The model under review builds one solid part; all positions refer to its coordinate system, in mm. A direction names the side the tool comes from. Coordinates: 2 decimals unless noted, no trailing zeros. Order: outer loops, then holes, each group sorted by start corner. A loop starts at its lowest first (then second) coordinate and runs counter-clockwise, first axis right, second up. Notation, with made-up numbers: (6.5, -30.5) -> (35.5, -30.5) arc R19 ccw to (35.5, 3.5) -> close; hole circle Ø8 at (24, -10.75). An arc over 180 degrees is marked (long way). Put each result on its own line as item: value.
from build123d import *

# Parameters (mm, degrees)
SKETCH1_R      = 11
EXTRUDE1_DEPTH = 3
SKETCH2_R      = 9
EXTRUDE2_DEPTH = 1.5
SKETCH3_R      = 7
EXTRUDE3_DEPTH = 1.5
SKETCH4_R      = 5
EXTRUDE4_DEPTH = 1.5
SKETCH5_R      = 3
EXTRUDE5_DEPTH = 1.5


with BuildPart() as part:
    # Sketch1 → Extrude1 (new body)
    with BuildSketch(Plane.XY):
        Circle(SKETCH1_R)
        with BuildLine():
            Line((2.224859546, 4.7), (-2.224859546, 4.7))
            ThreePointArc((-2.224859546, 4.7), (-3.676955262, 3.676955262), (-4.7, 2.224859546))
            Line((-4.7, 2.224859546), (-4.7, -2.224859546))
            ThreePointArc((-4.7, -2.224859546), (-3.676955262, -3.676955262), (-2.224859546, -4.7))
            Line((-2.224859546, -4.7), (2.224859546, -4.7))
            ThreePointArc((2.224859546, -4.7), (3.676955262, -3.676955262), (4.7, -2.224859546))
            Line((4.7, -2.224859546), (4.7, 2.224859546))
            ThreePointArc((4.7, 2.224859546), (3.676955262, 3.676955262), (2.224859546, 4.7))
        make_face(mode=Mode.SUBTRACT)
    extrude(amount=-EXTRUDE1_DEPTH)

    # Sketch2 → Extrude2 (add)
    with BuildSketch(Plane.XY):
        Circle(SKETCH2_R)
    extrude(amount=EXTRUDE2_DEPTH)

    # Sketch3 → Extrude3 (add)
    with BuildSketch(Plane.XY.offset(1.5)):
        Circle(SKETCH3_R)
    extrude(amount=EXTRUDE3_DEPTH)

    # Sketch4 → Extrude4 (add)
    with BuildSketch(Plane.XY.offset(3)):
        Circle(SKETCH4_R)
    extrude(amount=EXTRUDE4_DEPTH)

    # Sketch5 → Extrude5 (add)
    with BuildSketch(Plane.XY.offset(4.5)):
        Circle(SKETCH5_R)
    extrude(amount=EXTRUDE5_DEPTH)


solid = part.part
Item 1: For line 1 (Y direction, x = -4, z = 3.75); line 2 (Z direction, x = 2.5, y = 2); line 3 (Z direction, x = -2.5, y = 0.25), list the stretches that pass through material, from the lowest coordinate up. Write a range as from..to.
Answers below:
line 1: -3..3
line 2: 0..4.5
line 3: 0..6
Item 2: Consider section B-B on y = 0. Write out the cut boundary in (x, z), and give its area (3 significant figures).
Answers below:
outline: (-11, -3) -> (-4.7, -3) -> (-4.7, 0) -> (4.7, 0) -> (4.7, -3) -> (11, -3) -> (11, 0) -> (9, 0) -> (9, 1.5) -> (7, 1.5) -> (7, 3) -> (5, 3) -> (5, 4.5) -> (3, 4.5) -> (3, 6) -> (-3, 6) -> (-3, 4.5) -> (-5, 4.5) -> (-5, 3) -> (-7, 3) -> (-7, 1.5) -> (-9, 1.5) -> (-9, 0) -> (-11, 0) -> close
area: 110 mm^2
Item 3: Mouldability with a two-part tool opening along X and no side actions: class faces 4 (the flat face through (0, -7.3, 1.5)), 5 (the flat face through (4.7, 0, -1)), 6 (the flat face through (-4.7, 0, -1)), 7 (the cylindrical face through (-3, 0, 5)) as +X half, -X half, draft (parallel to the pull), parting line (faces both ways), or undercut.
Answers below:
face 4: draft
face 5: undercut
face 6: undercut
face 7: parting line
Item 4: Consider section D-D on z = 3.75. Write out the cut boundary in (x, y), and give its area (3 significant figures).
Answers below:
outline: circle Ø10 at (0, 0)
area: 78.5 mm^2
Item 5: For faces 1 (the flat face through (0, 0, 6)), 2 (the flat face through (0, 0, 0)), 3 (the flat face through (-0.1, -3.3, 4.5)), list the 3-axis set-ups (+Z, -Z, +X, -X, +Y, -Y) from which the entire face can be reached by the end or side of a thin tool; tool diameter is ignored.
Answers below:
face 1: +Z, +X, -X, +Y, -Y
face 2: -Z
face 3: +Z
Item 6: For pin 1 Ø6 at (x, y) = (-8.5, -3.5) entering from +Z; pin 2 Ø2 at (x, y) = (-8.5, -1) entering from +Z; pin 3 Ø1.5 at (y, z) = (-5.5, -0.5) entering from -X, all flat-tipped, find the tip position at first contact; note any pin that passes through.
Answers below:
pin 1: z = 3
pin 2: z = 1.5
pin 3: x = -9.92
Item 7: Consider section A-A on z = -2.25. Write out the cut boundary in (x, y), and give its area (3 significant figures).
Answers below:
outline: circle Ø22 at (0, 0); hole (-4.7, -2.22) arc R5.2 ccw to (-2.22, -4.7) -> (2.22, -4.7) arc R5.2 ccw to (4.7, -2.22) -> (4.7, 2.22) arc R5.2 ccw to (2.22, 4.7) -> (-2.22, 4.7) arc R5.2 ccw to (-4.7, 2.22) -> close
area: 301 mm^2
